The model under review builds one solid part; all positions refer to its coordinate system, in mm. Round coordinates to 2 decimals unless told otherwise and drop trailing zeros. Write each loop counter-clockwise with the first axis right and the second up, starting at its lowest first coordinate (ties: lowest second). Pieces come first, ordered by that corner, then holes. Notation, with made-up numbers: (-16.75, -22.5) -> (39.25, -22.5) arc R19 cw to (39.25, -0.5) -> close; hole circle Ø1 at (44, 2.25). An arc over 180 degrees is marked (long way). Answer in a Markdown table with one row per item. Add a question column.
```python
from build123d import *

# Parameters (mm, degrees)
BOSS_EXTRUDE1_DEPTH              = 3.175
F_1_4_0_25_DIAMETER_HOLE1_D      = 6.35
F_17_64_0_26563_DIAMETER_HOLE1_D = 6.747002
FILLET1_R                        = 2.54
F_1_4_0_25_DIAMETER_HOLE2_D      = 6.35


with BuildPart() as part:
    # Sketch1 → Boss-Extrude1 (new body)
    with BuildSketch(Plane.XY):
        Polygon((-1016, 514.35), (-1016, -50.8), (0, -50.8), (0, 0), align=None)
    extrude(amount=BOSS_EXTRUDE1_DEPTH)

    # 1/4 (0.25) Diameter Hole1 (through all)
    with Locations(Plane.XY.offset(3.175)):
        with Locations((-1003.3, 419.1), (-1003.3, 260.35), (-1003.3, 101.6)):
            Hole(F_1_4_0_25_DIAMETER_HOLE1_D / 2)

    # 17/64 (0.26563) Diameter Hole1 (through all)
    with Locations(Plane.XY.offset(3.175)):
        with Locations((-254, 19.05), (-711.2, 57.15), (-711.2, 19.05), (-254, 57.15)):
            Hole(F_17_64_0_26563_DIAMETER_HOLE1_D / 2)

    # Fillet1
    fillet1_edges = [part.edges().sort_by_distance(p)[0] for p in [
        (0, 0, 1.5875),
        (0, -50.8, 1.5875),
        (-1016, -50.8, 1.5875),
        (-1016, 514.35, 1.5875),
    ]]
    fillet(fillet1_edges, radius=FILLET1_R)

    # 1/4 (0.25) Diameter Hole2 (through all)
    with Locations(Plane.XY.offset(3.175)):
        with Locations((-913.865917768, 430.616531739), (-732.573803329, 338.837398804), (-188.697460012, 63.5), (-369.989574451, 155.279132935), (-551.28168889, 247.058265869)):
            Hole(F_1_4_0_25_DIAMETER_HOLE2_D / 2)


solid = part.part
```
1. Add section A-A on z = 1.8. State how many separate pieces and enclosed holes the cut face has, plus the area to 4 significant figures.
2. For L1, parallel to Y at x = -711.2, z = 1.7 (1 decimal); L2, parallel to Y at x = -254, z = 0.95; L3, parallel to X at y = 62, z = 0.35, list the stretches that pass through material, from the lowest coordinate up.
3. Add section B-B on x = -112. Write out the cut boundary in (y, z) (3 decimals), plus the area to 3 significant figures.
4. Add section C-C on y = 464. Write out the cut boundary in (x, z) (3 decimals).
Filled in:
| question | item | result |
|---|---|---|
| 1 | separate pieces | 1 |
| 1 | enclosed holes | 12 |
| 1 | area | 312,500 mm² |
| 2 | L1 | -50.8 to 15.7, 22.4 to 53.8, 60.5 to 360 |
| 2 | L2 | -50.8 to 15.68, 22.42 to 53.78, 60.52 to 128.59 |
| 2 | L3 | -1016 to -191.5, -185.9 to -122.47 |
| 3 | outline | (-50.8, 0) -> (56.7, 0) -> (56.7, 3.175) -> (-50.8, 3.175) -> close |
| 3 | area | 341 mm² |
| 4 | outline | (-1016, 0) -> (-916.543, 0) -> (-916.543, 3.175) -> (-1016, 3.175) -> close |
